```python
from build123d import *

# Parameters (mm, degrees)
SM_BASE_FLANGE_1_DEPTH            = 5
SM_EDGE_FLANGE_1_STRIP_W          = 26
SM_EDGE_FLANGE_1_STRIP_H          = 5
SM_EDGE_FLANGE_1_STRIP_CUT_DEPTH  = 45
SM_EDGE_FLANGE_1_RELIEF_W         = 28.5
SM_EDGE_FLANGE_1_RELIEF_H         = 2.5
SM_EDGE_FLANGE_1_RELIEF_CUT_DEPTH = 5
SM_EDGE_FLANGE_1_DEPTH            = 45
SM_EDGE_FLANGE_2_STRIP_W          = 26
SM_EDGE_FLANGE_2_STRIP_H          = 5
SM_EDGE_FLANGE_2_STRIP_CUT_DEPTH  = 45
SM_EDGE_FLANGE_2_RELIEF_W         = 28.5
SM_EDGE_FLANGE_2_RELIEF_H         = 2.5
SM_EDGE_FLANGE_2_RELIEF_CUT_DEPTH = 5
SM_EDGE_FLANGE_2_DEPTH            = 45
SM_EDGE_FLANGE_14_DEPTH           = 40
SM_EDGE_FLANGE_15_DEPTH           = 40
SM_EDGE_FLANGE_16_DEPTH           = 40
SM_EDGE_FLANGE_17_DEPTH           = 40
SM_EDGE_FLANGE_18_STRIP_W         = 26
SM_EDGE_FLANGE_18_STRIP_H         = 5
SM_EDGE_FLANGE_18_STRIP_CUT_DEPTH = 40
SM_EDGE_FLANGE_18_DEPTH           = 40
SM_EDGE_FLANGE_19_STRIP_W         = 26
SM_EDGE_FLANGE_19_STRIP_H         = 5
SM_EDGE_FLANGE_19_STRIP_CUT_DEPTH = 40
SM_EDGE_FLANGE_19_DEPTH           = 40
SM_EDGE_FLANGE_20_STRIP_W         = 26
SM_EDGE_FLANGE_20_STRIP_H         = 5
SM_EDGE_FLANGE_20_STRIP_CUT_DEPTH = 40
SM_EDGE_FLANGE_20_DEPTH           = 40
SM_EDGE_FLANGE_21_STRIP_W         = 26
SM_EDGE_FLANGE_21_STRIP_H         = 5
SM_EDGE_FLANGE_21_STRIP_CUT_DEPTH = 40
SM_EDGE_FLANGE_21_DEPTH           = 40
CUT_EXTRUDE_START                 = -35
SKETCH_80_R                       = 2.5
CUT_EXTRUDE_1_DEPTH               = 5
CUT_EXTRUDE_3_DEPTH               = 124.060960503
CUT_EXTRUDE_3_DEPTH_BACK          = 124.060960503
SKETCH_83_R                       = 2.5
CUT_EXTRUDE_START_2               = -30
SKETCH_84_R                       = 2.5
CUT_EXTRUDE_5_DEPTH               = 5


# Sheet-metal steps are written as plain solids
with BuildPart() as part:
    # Sketch 1 → 基体-法兰1 (new body)
    with BuildSketch(Plane(origin=(0, 0, 0), x_dir=(1, 0, 0), z_dir=(0, 1, 0))):
        Polygon((-25, -25), (-25, -50), (-50, -50), (-50, 50), (-25, 50), (-25, 25), (25, 25), (25, 50), (50, 50), (50, -50), (25, -50), (25, -25), align=None)
    extrude(amount=-SM_BASE_FLANGE_1_DEPTH)

    # 边线-法兰1 strip (across the edge) → 边线-法兰1 strip cut (cut)
    with BuildSketch(Plane(origin=(22.5, 0, -25), x_dir=(0, 0, 1), z_dir=(-1, 0, 0))):
        with Locations((-10, -2.5)):
            Rectangle(SM_EDGE_FLANGE_1_STRIP_W, SM_EDGE_FLANGE_1_STRIP_H)
    extrude(amount=SM_EDGE_FLANGE_1_STRIP_CUT_DEPTH, mode=Mode.SUBTRACT)

    # 边线-法兰1 relief (on the sheet) → 边线-法兰1 relief cut (cut)
    with BuildSketch(Plane(origin=(22.5, 0, -22), x_dir=(0, 0, 1), z_dir=(0, 1, 0))):
        with Locations((-11.75, 1.25)):
            Rectangle(SM_EDGE_FLANGE_1_RELIEF_W, SM_EDGE_FLANGE_1_RELIEF_H)
        with Locations((-11.75, -46.25)):
            Rectangle(SM_EDGE_FLANGE_1_RELIEF_W, SM_EDGE_FLANGE_1_RELIEF_H)
    extrude(amount=-SM_EDGE_FLANGE_1_RELIEF_CUT_DEPTH, mode=Mode.SUBTRACT)

    # 边线-法兰1 section (across the edge) → 边线-法兰1 (add)
    with BuildSketch(Plane(origin=(22.5, 0, -25), x_dir=(0, 0, 1), z_dir=(-1, 0, 0))):
        with BuildLine():
            Line((-5, 3), (-5, 70))
            Line((-5, 70), (0, 70))
            Line((0, 70), (0, 3))
            ThreePointArc((0, 3), (0.878679656, 0.878679656), (3, 0))
            Line((3, 0), (3, -5))
            ThreePointArc((3, -5), (-2.656854249, -2.656854249), (-5, 3))
        make_face()
    extrude(amount=SM_EDGE_FLANGE_1_DEPTH)

    # 边线-法兰2 strip (across the edge) → 边线-法兰2 strip cut (cut)
    with BuildSketch(Plane(origin=(-22.5, 0, 25), x_dir=(0, 0, -1), z_dir=(1, 0, 0))):
        with Locations((-10, -2.5)):
            Rectangle(SM_EDGE_FLANGE_2_STRIP_W, SM_EDGE_FLANGE_2_STRIP_H)
    extrude(amount=SM_EDGE_FLANGE_2_STRIP_CUT_DEPTH, mode=Mode.SUBTRACT)

    # 边线-法兰2 relief (on the sheet) → 边线-法兰2 relief cut (cut)
    with BuildSketch(Plane(origin=(-22.5, 0, 22), x_dir=(0, 0, -1), z_dir=(0, 1, 0))):
        with Locations((-11.75, 1.25)):
            Rectangle(SM_EDGE_FLANGE_2_RELIEF_W, SM_EDGE_FLANGE_2_RELIEF_H)
        with Locations((-11.75, -46.25)):
            Rectangle(SM_EDGE_FLANGE_2_RELIEF_W, SM_EDGE_FLANGE_2_RELIEF_H)
    extrude(amount=-SM_EDGE_FLANGE_2_RELIEF_CUT_DEPTH, mode=Mode.SUBTRACT)

    # 边线-法兰2 section (across the edge) → 边线-法兰2 (add)
    with BuildSketch(Plane(origin=(-22.5, 0, 25), x_dir=(0, 0, -1), z_dir=(1, 0, 0))):
        with BuildLine():
            Line((-5, 3), (-5, 70))
            Line((-5, 70), (0, 70))
            Line((0, 70), (0, 3))
            ThreePointArc((0, 3), (0.878679656, 0.878679656), (3, 0))
            Line((3, 0), (3, -5))
            ThreePointArc((3, -5), (-2.656854249, -2.656854249), (-5, 3))
        make_face()
    extrude(amount=SM_EDGE_FLANGE_2_DEPTH)

    # 边线-法兰14 section (across the edge) → 边线-法兰14 (add)
    with BuildSketch(Plane(origin=(53, -5, 10), x_dir=(-1, 0, 0), z_dir=(0, 0, 1))):
        with BuildLine():
            Line((-5, 3), (-5, 30))
            Line((-5, 30), (0, 30))
            Line((0, 30), (0, 3))
            ThreePointArc((0, 3), (0.878679656, 0.878679656), (3, 0))
            Line((3, 0), (3, -5))
            ThreePointArc((3, -5), (-2.656854249, -2.656854249), (-5, 3))
        make_face()
    extrude(amount=SM_EDGE_FLANGE_14_DEPTH)

    # 边线-法兰15 section (across the edge) → 边线-法兰15 (add)
    with BuildSketch(Plane(origin=(53, -5, -50), x_dir=(-1, 0, 0), z_dir=(0, 0, 1))):
        with BuildLine():
            Line((-5, 3), (-5, 30))
            Line((-5, 30), (0, 30))
            Line((0, 30), (0, 3))
            ThreePointArc((0, 3), (0.878679656, 0.878679656), (3, 0))
            Line((3, 0), (3, -5))
            ThreePointArc((3, -5), (-2.656854249, -2.656854249), (-5, 3))
        make_face()
    extrude(amount=SM_EDGE_FLANGE_15_DEPTH)

    # 边线-法兰16 section (across the edge) → 边线-法兰16 (add)
    with BuildSketch(Plane(origin=(-53, -5, -10), x_dir=(1, 0, 0), z_dir=(0, 0, -1))):
        with BuildLine():
            Line((-5, 3), (-5, 30))
            Line((-5, 30), (0, 30))
            Line((0, 30), (0, 3))
            ThreePointArc((0, 3), (0.878679656, 0.878679656), (3, 0))
            Line((3, 0), (3, -5))
            ThreePointArc((3, -5), (-2.656854249, -2.656854249), (-5, 3))
        make_face()
    extrude(amount=SM_EDGE_FLANGE_16_DEPTH)

    # 边线-法兰17 section (across the edge) → 边线-法兰17 (add)
    with BuildSketch(Plane(origin=(-53, -5, 50), x_dir=(1, 0, 0), z_dir=(0, 0, -1))):
        with BuildLine():
            Line((-5, 3), (-5, 30))
            Line((-5, 30), (0, 30))
            Line((0, 30), (0, 3))
            ThreePointArc((0, 3), (0.878679656, 0.878679656), (3, 0))
            Line((3, 0), (3, -5))
            ThreePointArc((3, -5), (-2.656854249, -2.656854249), (-5, 3))
        make_face()
    extrude(amount=SM_EDGE_FLANGE_17_DEPTH)

    # 边线-法兰18 strip (across the edge) → 边线-法兰18 strip cut (cut)
    with BuildSketch(Plane(origin=(-58, -35, -50), x_dir=(0, 1, 0), z_dir=(0, 0, 1))):
        with Locations((-5, -2.5)):
            Rectangle(SM_EDGE_FLANGE_18_STRIP_W, SM_EDGE_FLANGE_18_STRIP_H)
    extrude(amount=SM_EDGE_FLANGE_18_STRIP_CUT_DEPTH, mode=Mode.SUBTRACT)

    # 边线-法兰18 section (across the edge) → 边线-法兰18 (add)
    with BuildSketch(Plane(origin=(-58, -35, -50), x_dir=(0, 1, 0), z_dir=(0, 0, 1))):
        with BuildLine():
            Line((0, 3), (0, 30))
            Line((0, 30), (5, 30))
            Line((5, 30), (5, 3))
            ThreePointArc((5, 3), (5.878679656, 0.878679656), (8, 0))
            Line((8, 0), (8, -5))
            ThreePointArc((8, -5), (2.343145751, -2.656854249), (0, 3))
        make_face()
    extrude(amount=SM_EDGE_FLANGE_18_DEPTH)

    # 边线-法兰19 strip (across the edge) → 边线-法兰19 strip cut (cut)
    with BuildSketch(Plane(origin=(-58, -35, 10), x_dir=(0, 1, 0), z_dir=(0, 0, 1))):
        with Locations((-5, -2.5)):
            Rectangle(SM_EDGE_FLANGE_19_STRIP_W, SM_EDGE_FLANGE_19_STRIP_H)
    extrude(amount=SM_EDGE_FLANGE_19_STRIP_CUT_DEPTH, mode=Mode.SUBTRACT)

    # 边线-法兰19 section (across the edge) → 边线-法兰19 (add)
    with BuildSketch(Plane(origin=(-58, -35, 10), x_dir=(0, 1, 0), z_dir=(0, 0, 1))):
        with BuildLine():
            Line((0, 3), (0, 30))
            Line((0, 30), (5, 30))
            Line((5, 30), (5, 3))
            ThreePointArc((5, 3), (5.878679656, 0.878679656), (8, 0))
            Line((8, 0), (8, -5))
            ThreePointArc((8, -5), (2.343145751, -2.656854249), (0, 3))
        make_face()
    extrude(amount=SM_EDGE_FLANGE_19_DEPTH)

    # 边线-法兰20 strip (across the edge) → 边线-法兰20 strip cut (cut)
    with BuildSketch(Plane(origin=(58, -35, 50), x_dir=(0, 1, 0), z_dir=(0, 0, -1))):
        with Locations((-5, -2.5)):
            Rectangle(SM_EDGE_FLANGE_20_STRIP_W, SM_EDGE_FLANGE_20_STRIP_H)
    extrude(amount=SM_EDGE_FLANGE_20_STRIP_CUT_DEPTH, mode=Mode.SUBTRACT)

    # 边线-法兰20 section (across the edge) → 边线-法兰20 (add)
    with BuildSketch(Plane(origin=(58, -35, 50), x_dir=(0, 1, 0), z_dir=(0, 0, -1))):
        with BuildLine():
            Line((0, 3), (0, 30))
            Line((0, 30), (5, 30))
            Line((5, 30), (5, 3))
            ThreePointArc((5, 3), (5.878679656, 0.878679656), (8, 0))
            Line((8, 0), (8, -5))
            ThreePointArc((8, -5), (2.343145751, -2.656854249), (0, 3))
        make_face()
    extrude(amount=SM_EDGE_FLANGE_20_DEPTH)

    # 边线-法兰21 strip (across the edge) → 边线-法兰21 strip cut (cut)
    with BuildSketch(Plane(origin=(58, -35, -10), x_dir=(0, 1, 0), z_dir=(0, 0, -1))):
        with Locations((-5, -2.5)):
            Rectangle(SM_EDGE_FLANGE_21_STRIP_W, SM_EDGE_FLANGE_21_STRIP_H)
    extrude(amount=SM_EDGE_FLANGE_21_STRIP_CUT_DEPTH, mode=Mode.SUBTRACT)

    # 边线-法兰21 section (across the edge) → 边线-法兰21 (add)
    with BuildSketch(Plane(origin=(58, -35, -10), x_dir=(0, 1, 0), z_dir=(0, 0, -1))):
        with BuildLine():
            Line((0, 3), (0, 30))
            Line((0, 30), (5, 30))
            Line((5, 30), (5, 3))
            ThreePointArc((5, 3), (5.878679656, 0.878679656), (8, 0))
            Line((8, 0), (8, -5))
            ThreePointArc((8, -5), (2.343145751, -2.656854249), (0, 3))
        make_face()
    extrude(amount=SM_EDGE_FLANGE_21_DEPTH)

    # 草图80 → 切除-拉伸1 (cut)
    with BuildSketch(Plane(origin=(0, 0, 0), x_dir=(1, 0, 0), z_dir=(0, 1, 0)).offset(CUT_EXTRUDE_START)):
        with Locations(Location((-75, 40, 0), (0, 0, 270))):
            Circle(SKETCH_80_R)
        with Locations(Location((75, 40, 0), (0, 0, 270))):
            Circle(SKETCH_80_R)
        with Locations(Location((-75, -40, 0), (0, 0, 270))):
            Circle(SKETCH_80_R)
        with Locations(Location((75, -40, 0), (0, 0, 270))):
            Circle(SKETCH_80_R)
    extrude(amount=CUT_EXTRUDE_1_DEPTH, mode=Mode.SUBTRACT)

    # 草图83 → 切除-拉伸3 (cut, two sides: drawn at the far end of the back side and taken through both)
    with BuildSketch(Plane.XY.offset(-CUT_EXTRUDE_3_DEPTH_BACK)):
        with Locations((0, 50)):
            Circle(SKETCH_83_R)
        with Locations((0, 30)):
            Circle(SKETCH_83_R)
    extrude(amount=CUT_EXTRUDE_3_DEPTH + CUT_EXTRUDE_3_DEPTH_BACK, mode=Mode.SUBTRACT)

    # 草图84 → 切除-拉伸5 (cut)
    with BuildSketch(Plane(origin=(0, 0, 0), x_dir=(1, 0, 0), z_dir=(0, 1, 0)).offset(CUT_EXTRUDE_START_2)):
        with Locations(Location((75, 22.5, 0), (0, 0, 270))):
            Circle(SKETCH_84_R)
        with Locations(Location((75, -22.5, 0), (0, 0, 270))):
            Circle(SKETCH_84_R)
        with Locations(Location((-75, -22.5, 0), (0, 0, 270))):
            Circle(SKETCH_84_R)
        with Locations(Location((-75, 22.5, 0), (0, 0, 270))):
            Circle(SKETCH_84_R)
    extrude(amount=-CUT_EXTRUDE_5_DEPTH, mode=Mode.SUBTRACT)


solid = part.part
```
Part model, mm, in its own coordinate system. A direction names the side the tool comes from. Round coordinates to 2 decimals unless told otherwise and drop trailing zeros. Loops run counter-clockwise (first coordinate to the right, second up) from the corner with the lowest first, then second, coordinate; pieces in that order, holes last.
Item 1: Cut at C-C, the plane z = 35.5. Give the cut face in (x, y), then the cut area to 3 significant figures.
Item 2: Cut at B-B, the plane x = 64. Give the cut face in (y, z), then the cut area to 3 significant figures.
Item 3: Cut at D-D, the plane x = 0. Give the cut face in (y, z).
Item 4: Cut at A-A, the plane y = 50. Give the cut face in (x, z).
Item 5: Mould opens along X. For faces 6 (the face through (57.8, -23.9, 10)), 7 (the face through (-53, -18, -30)), 8 (the face through (-58, -17, -30)) say: +X half, -X half, draft (parallel to the pull), parting line (faces both ways), or undercut.
Item 6: Drill centre lines: line 1 (Z direction, x = 3.5, y = 47.5); line 2 (X direction, y = -33, z = -22); line 3 (X direction, y = 30, z = -28.85). Where is each one in solid material? Low to high.
Item 7: Drop flat-ended pins along their axis: P1, Ø1.5, axis at x = -6, y = 41, coming from the +Z side; P2, Ø13.5, axis at x = 6.5, y = 21.5, coming from the -Z side; P3, Ø5.5, axis at y = -18, z = 21, coming from the +X side. Give the stop position or say it passes through.
Item 8: 3-axis set-ups, long thin cutter, end or side, ignore diameter. For faces 1 (the face through (53, -18, -30)), 2 (the face through (0, 37, 25)), 3 (the face through (-22.5, 33, 27)), 4 (the face through (25, -2, -35)), 5 (the face through (-0.315, -2.719, 27.594)): which of +Z, -Z, +X, -X, +Y, -Y reach the whole face in a straight line?
A:
1. outline: (-88, -35) - (-61, -35) arc R8 ccw to (-53, -27) - (-53, -8) arc R3 cw to (-50, -5) - (-25, -5) - (-25, 0) - (-50, 0) arc R8 ccw to (-58, -8) - (-58, -27) arc R3 cw to (-61, -30) - (-88, -30) - close; (25, -5) - (50, -5) arc R3 cw to (53, -8) - (53, -27) arc R8 ccw to (61, -35) - (88, -35) - (88, -30) - (61, -30) arc R3 cw to (58, -27) - (58, -8) arc R8 ccw to (50, 0) - (25, 0) - close
1. area: 883 mm2
2. outline: (-35, -50) - (-30, -50) - (-30, -10) - (-35, -10) - close; (-35, 10) - (-30, 10) - (-30, 50) - (-35, 50) - close
2. area: 400 mm2
3. outline: (-5, -22) arc R8 ccw to (3, -30) - (27.5, -30) - (27.5, -25) - (3, -25) arc R3 cw to (0, -22) - (0, 22) arc R3 cw to (3, 25) - (27.5, 25) - (27.5, 30) - (3, 30) arc R8 ccw to (-5, 22) - close; (32.5, -30) - (47.5, -30) - (47.5, -25) - (32.5, -25) - close; (32.5, 25) - (47.5, 25) - (47.5, 30) - (32.5, 30) - close; (52.5, -30) - (70, -30) - (70, -25) - (52.5, -25) - close; (52.5, 25) - (70, 25) - (70, 30) - (52.5, 30) - close
4. outline: (-22.5, -30) - (-2.5, -30) - (-2.5, -25) - (-22.5, -25) - close; (-22.5, 25) - (-2.5, 25) - (-2.5, 30) - (-22.5, 30) - close; (2.5, -30) - (22.5, -30) - (22.5, -25) - (2.5, -25) - close; (2.5, 25) - (22.5, 25) - (22.5, 30) - (2.5, 30) - close
5. face 6: draft
5. face 7: undercut
5. face 8: -X half
6. line 1: z = -30 to -25, 25 to 30
6. line 2: x = -88 to -77.45, -72.55 to -55.71, 55.71 to 72.55, 77.45 to 88
6. line 3: x = -22.5 to -2.5, 2.5 to 22.5
7. P1: stops at z = 30
7. P2: stops at z = -30
7. P3: stops at x = 58
8. face 1: +Z, -Z, -Y
8. face 2: +X, -X, +Y
8. face 3: +Z, +Y, -Y
8. face 4: -Z, +Y, -Y
8. face 5: +Z, -Y
